The drawing under review shows one solid part. Ordinate dimensions are in mm from its lowest x, y, z. A direction names the side the tool comes from. Coordinates: 2 decimals unless noted, no trailing zeros. Write each loop counter-clockwise with the first axis right and the second up, starting at its lowest first coordinate (ties: lowest second). Pieces come first, ordered by that corner, then holes. Notation, with made-up numbers: (-12, 55.5) -> (-7, 55.5) arc R33 cw to (-7, 86.5) -> close; hole circle Ø6 at (73, 62). An arc over 180 degrees is marked (long way). One line per item, written item: value. Start each with the question number.
1) For probe 1 along Z at (x, y) = (10.75, 0.35); probe 2 along X at (y, z) = (3.25, 10.5); probe 3 along X at (y, z) = (4.2, 14), list the stretches that pass through material, from the lowest coordinate up. Write a range as from..to.
2) Add section A-A (x = 10.5). State the section outline as (y, z) points, and give its area (3 significant figures).
3) Mouldability with a two-part tool opening along X and no side actions: class the marked faces 3, 4 and 5 as released by +X, released by -X, zero draft, split by the parting line, or undercut.
4) Add section D-D (z = 18.75). State the section outline as (x, y) points.
5) For pin 1 Ø3 at (x, z) = (3.5, 13) entering from -Y; pin 2 Ø7 at (x, z) = (10.5, 10.5) entering from +Y; pin 3 Ø1.5 at (x, y) = (9, 2) entering from +Z; pin 4 Ø1.5 at (x, y) = (15, 3.5) entering from -Z, all flat-tipped, find the tip position at first contact; note any pin that passes through.
6) Add section C-C (y = 3.1). State the section outline as (x, z) points, and give its area (3 significant figures).
7) Machinability: for the marked faces 1 and 2, which of the approach directions +Z, -Z, +X, -X, +Y, -Y give a long, thin tool a straight path to every point of the face, cutting with its end or side? Answer none if there is none.
8) Add section B-B (z = 10.5). State the section outline as (x, y) points, and give its area (3 significant figures).
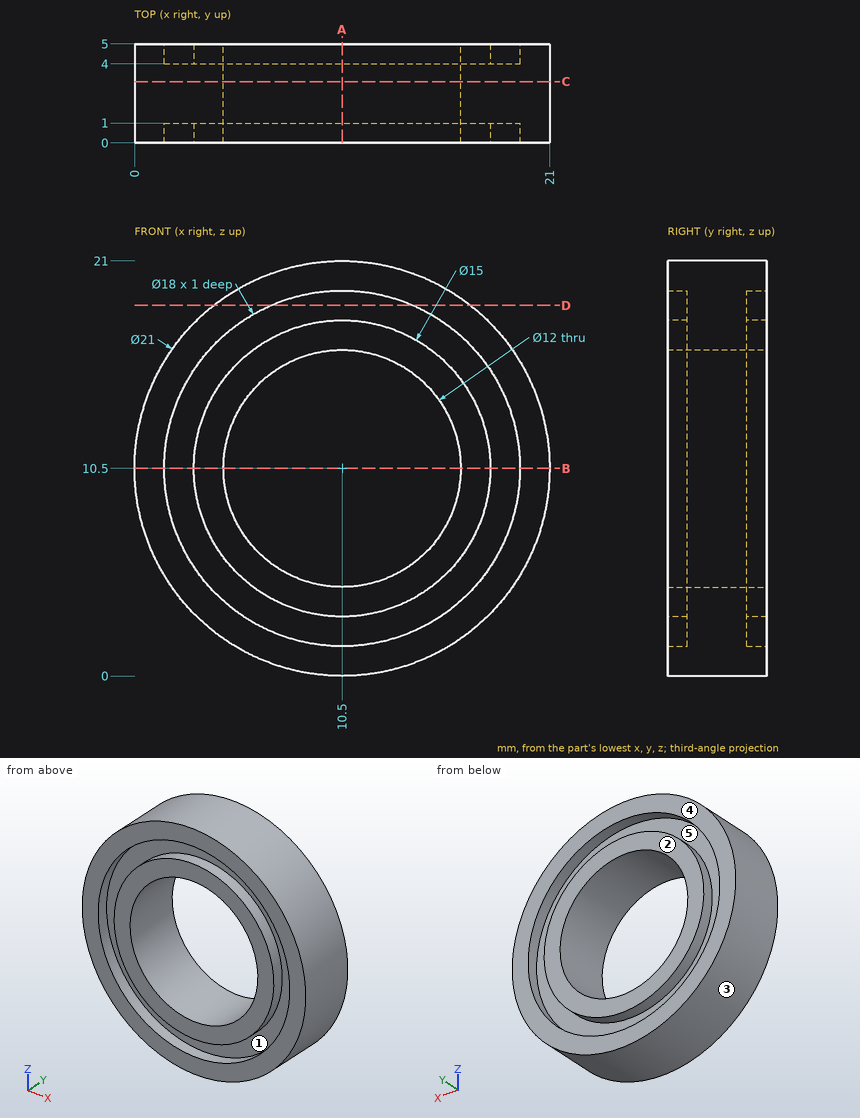
Numbers:
1. probe 1: 0..1.5, 3..4.51, 16.49..18, 19.5..21
1. probe 2: 0..4.5, 16.5..21
1. probe 3: 0.6..2.21, 3.87..5.63, 15.37..17.13, 18.79..20.4
2. outline: (0, 0) -> (5, 0) -> (5, 1.5) -> (4, 1.5) -> (4, 3) -> (5, 3) -> (5, 4.5) -> (0, 4.5) -> (0, 3) -> (1, 3) -> (1, 1.5) -> (0, 1.5) -> close; (0, 16.5) -> (5, 16.5) -> (5, 18) -> (4, 18) -> (4, 19.5) -> (5, 19.5) -> (5, 21) -> (0, 21) -> (0, 19.5) -> (1, 19.5) -> (1, 18) -> (0, 18) -> close
2. area: 39.0 mm²
3. face 3: split by the parting line
3. face 4: zero draft
3. face 5: undercut
4. outline: (4, 0) -> (6.9, 0) -> (6.9, 1) -> (14.1, 1) -> (14.1, 0) -> (17, 0) -> (17, 5) -> (14.1, 5) -> (14.1, 4) -> (6.9, 4) -> (6.9, 5) -> (4, 5) -> close
5. pin 1: y = 0
5. pin 2: through
5. pin 3: z = 20.97
5. pin 4: z = 0.69
6. outline: circle Ø21 at (10.5, 10.5); hole circle Ø12 at (10.5, 10.5)
6. area: 233 mm²
7. face 1: -Y
7. face 2: +Z, -Z, +X, -X, +Y
8. outline: (0, 0) -> (1.5, 0) -> (1.5, 1) -> (3, 1) -> (3, 0) -> (4.5, 0) -> (4.5, 5) -> (3, 5) -> (3, 4) -> (1.5, 4) -> (1.5, 5) -> (0, 5) -> close; (16.5, 0) -> (18, 0) -> (18, 1) -> (19.5, 1) -> (19.5, 0) -> (21, 0) -> (21, 5) -> (19.5, 5) -> (19.5, 4) -> (18, 4) -> (18, 5) -> (16.5, 5) -> close
8. area: 39.0 mm²
